Can you work these out from the model? Positions are in its coordinate system, mm. A direction names the side the tool comes from. Round coordinates to 2 decimals unless told otherwise and drop trailing zeros. Order: outer loops, then holes, each group sorted by start corner. A loop starts at its lowest first (then second) coordinate and runs counter-clockwise, first axis right, second up.
from build123d import *

# Parameters (mm, degrees)
SALIENTE_EXTRUIR1_DEPTH = 50
REDONDEO1_R             = 15
CROQUIS2_R              = 7.5
CORTAR_EXTRUIR1_DEPTH   = 30
REDONDEO3_R             = 25
CROQUIS3_R              = 7.5
CORTAR_EXTRUIR2_DEPTH   = 7.5


with BuildPart() as part:
    # Croquis1 → Saliente-Extruir1 (new body)
    with BuildSketch(Plane.XY):
        Polygon((0, 0), (30, 0), (30, -40), (40, -40), (40, -80), (-10, -80), (-10, -40), (0, -40), align=None)
    extrude(amount=SALIENTE_EXTRUIR1_DEPTH)

    # Redondeo1
    redondeo1_edges = [part.edges().sort_by_distance(p)[0] for p in [
        (15, 0, 0),
        (15, 0, 50),
    ]]
    fillet(redondeo1_edges, radius=REDONDEO1_R)

    # Croquis2 → Cortar-Extruir1 (cut)
    with BuildSketch(Plane(origin=(30, 0, 0), x_dir=(0, 0, -1), z_dir=(1, 0, 0))):
        with Locations(Location((-25, -15, 0), (0, 0, 90))):
            Circle(CROQUIS2_R)
    extrude(amount=-CORTAR_EXTRUIR1_DEPTH, mode=Mode.SUBTRACT)

    # Redondeo3
    # the kernel refuses this fillet: 25 mm, written as the material it takes off along each edge
    with BuildSketch(Plane(origin=(-10, -142.5, 50), x_dir=(1, 0, 0), z_dir=(0, 1, 0)), Plane(origin=(40, 22.5, 50), x_dir=(-1, 0, 0), z_dir=(0, -1, 0))) as redondeo3_piece_1:
        with BuildLine():
            CenterArc((REDONDEO3_R, REDONDEO3_R), REDONDEO3_R, 180, 90)
            Line((0, REDONDEO3_R), (0, 0))
            Line((0, 0), (REDONDEO3_R, 0))
        make_face()
    extrude(amount=165, mode=Mode.SUBTRACT)
    with BuildSketch(Plane(origin=(-10, -142.5, 0), x_dir=(1, 0, 0), z_dir=(0, 1, 0)), Plane(origin=(40, 22.5, 0), x_dir=(-1, 0, 0), z_dir=(0, -1, 0))) as redondeo3_piece_2:
        with BuildLine():
            CenterArc((REDONDEO3_R, -REDONDEO3_R), REDONDEO3_R, 90, 90)
            Line((0, -REDONDEO3_R), (0, 0))
            Line((0, 0), (REDONDEO3_R, 0))
        make_face()
    extrude(amount=165, mode=Mode.SUBTRACT)

    # Croquis3 → Cortar-Extruir2 (cut)
    with BuildSketch(Plane.XZ.offset(80)):
        with Locations(Location((15, 25, 0), (0, 0, 270))):
            Circle(CROQUIS3_R)
    extrude(amount=-CORTAR_EXTRUIR2_DEPTH, mode=Mode.SUBTRACT)


solid = part.part
(1) I'm going to push flat-ended pins straight in: pin 1 Ø5 at (x, y) = (33.5, -67) entering from -Z; pin 2 Ø8 at (y, z) = (-42.5, 12.5) entering from +X; pin 3 Ø13.5 at (y, z) = (-15, 25) entering from -X; pin 4 Ø2 at (x, y) = (7.5, -11) entering from +Z. Where does each tip first touch, or does it pass through?
(2) I want a section at C-C, the plane x = 15. List the corners of the cut face in (y, z) for me.
(3) On a 3-axis mill with a long thin cutter (end or side, diameter ignored), from which of +Z, -Z, +X, -X, +Y, -Y can I reach the whole of each face in a straight line? I mean faces 5 (the face through (30, -24, 25)), 6 (the face through (24.58, -50.91, 1.91)), 7 (the face through (15, -72.5, 25)). Say none if no direction works.
(4) I want a section at A-A, the plane z = 25. List the corners of the cut face in (x, y) for me, plus the area to 3 significant figures.
(5) Please list where these lines run through material, in increasing order: probe 1 along X at (y, z) = (-76, 25); probe 2 along Y at (x, z) = (-1, 16.5); probe 3 along Y at (x, z) = (21, 25.5).
(6) If we mould it in two halves opening along Y, with no side actions, what happens to faces 1 (the face through (15.2, -20.5, 30.1)), 2 (the face through (21, -80, 30)), 3 (the face through (0, -25, 25)), 4 (the face through (-4, -40, 25))? For each: pulls with the +Y half, pulls with the -Y half, needs draft (parallel to the pull), parting line crosses it, or undercut.
(7) I want a section at D-D, the plane z = 30.5. List the corners of the cut face in (x, y) for me.
(8) I want a section at B-B, the plane y = -12.5. List the corners of the cut face in (x, z) for me, plus the area to 3 significant figures.
Ans:
1. pin 1: stops at z = 5.79
1. pin 2: stops at x = 38.51
1. pin 3: passes through
1. pin 4: stops at z = 49.14
2. outline: (-80, 0) - (-15, 0) arc R15 ccw to (0, 15) - (0, 35) arc R15 ccw to (-15, 50) - (-80, 50) - (-80, 32.5) - (-72.5, 32.5) - (-72.5, 17.5) - (-80, 17.5) - close; hole circle Ø15 at (-15, 25)
3. face 5: +Z, -Z, +X, +Y
3. face 6: +Y, -Y
3. face 7: -Y
4. outline: (-10, -80) - (7.5, -80) - (7.5, -72.5) - (22.5, -72.5) - (22.5, -80) - (40, -80) - (40, -40) - (30, -40) - (30, -22.5) - (0, -22.5) - (0, -40) - (-10, -40) - close; (0, -7.5) - (30, -7.5) - (30, 0) - (0, 0) - close
4. area: 2,640 mm2
5. probe 1: x = -10 to 7.5, 22.5 to 40
5. probe 2: y = -80 to -40
5. probe 3: y = -72.5 to -22.48, -7.52 to 0
6. face 1: undercut
6. face 2: pulls with the -Y half
6. face 3: needs draft
6. face 4: pulls with the +Y half
7. outline: (-9.39, -80) - (9.9, -80) - (9.9, -72.5) - (20.1, -72.5) - (20.1, -80) - (39.39, -80) - (39.39, -40) - (30, -40) - (30, -20.1) - (0, -20.1) - (0, -40) - (-9.39, -40) - close; (0, -9.9) - (30, -9.9) - (30, 0) - (0, 0) - close
8. outline: (0, 5) arc R25 ccw to (11.77, 0.21) - (18.23, 0.21) arc R25 ccw to (30, 5) - (30, 17.93) - (0, 17.93) - close; (0, 32.07) - (30, 32.07) - (30, 45) arc R25 ccw to (18.23, 49.79) - (11.77, 49.79) arc R25 ccw to (0, 45) - close
8. area: 978 mm2
